```python
from build123d import *

# Parameters (mm, degrees)
F1_DEPTH = 22.5
F2_DEPTH = 8.5
F0_W     = 10
F0_H     = 50
F3_DEPTH = 17
F6_DEPTH = 14
F7_DEPTH = 18


with BuildPart() as f1:
    # F0 (on Front) → F1 (new body, symmetric)
    with BuildSketch(Plane.XZ):
        with BuildLine():
            Line((0, 15), (0, 25))
            ThreePointArc((0, 25), (-25, 0), (0, -25))
            Line((0, -25), (0, -15))
            ThreePointArc((0, -15), (-15, 0), (0, 15))
        make_face()
        with BuildLine():
            ThreePointArc((0, -25), (17.6776695297, -17.6776695297), (25, 0))
            ThreePointArc((25, 0), (17.6776695297, 17.6776695297), (0, 25))
            Line((0, 25), (0, 15))
            ThreePointArc((0, 15), (10.6066017178, 10.6066017178), (15, 0))
            ThreePointArc((15, 0), (10.6066017178, -10.6066017178), (0, -15))
            Line((0, -15), (0, -25))
        make_face()
    extrude(amount=F1_DEPTH, both=True)

    # F0 (on Front) → F2 (join, symmetric)
    with BuildSketch(Plane.XZ):
        with BuildLine():
            ThreePointArc((0, 25), (17.6776695297, 17.6776695297), (25, 0))
            ThreePointArc((25, 0), (17.6776695297, -17.6776695297), (0, -25))
            Line((0, -25), (70, -25))
            Line((70, -25), (70, 25))
            Line((70, 25), (0, 25))
        make_face()
    extrude(amount=F2_DEPTH, both=True)

    # F0 (on Front) → F3 (join, symmetric)
    with BuildSketch(Plane.XZ):
        with Locations((75, 0)):
            Rectangle(F0_W, F0_H)
    extrude(amount=F3_DEPTH, both=True)

    # F5 (on offset) → F6 (join)
    with BuildSketch(Plane.XZ.offset(17)):
        with BuildLine():
            Line((93.4168760482, 25), (70, 25))
            Line((70, 25), (70, -25))
            Line((70, -25), (93.4168760482, -25))
            ThreePointArc((93.4168760482, -25), (80, 0), (93.4168760482, 25))
        make_face()
    extrude(amount=F6_DEPTH)

    # F5 (on offset) → F7 (join)
    with BuildSketch(Plane.XZ.offset(17)):
        with BuildLine():
            Line((110, 25), (93.4168760482, 25))
            ThreePointArc((93.4168760482, 25), (80, 0), (93.4168760482, -25))
            Line((93.4168760482, -25), (110, -25))
            Line((110, -25), (110, -15))
            ThreePointArc((110, -15), (95, 0), (110, 15))
            Line((110, 15), (110, 25))
        make_face()
        with BuildLine():
            ThreePointArc((140, 0), (124.1863716546, 26.4338203685), (93.4168760482, 25))
            Line((93.4168760482, 25), (110, 25))
            Line((110, 25), (110, 15))
            ThreePointArc((110, 15), (120.6066017178, 10.6066017178), (125, 0))
            ThreePointArc((125, 0), (120.6066017178, -10.6066017178), (110, -15))
            Line((110, -15), (110, -25))
            Line((110, -25), (93.4168760482, -25))
            ThreePointArc((93.4168760482, -25), (124.1863716546, -26.4338203685), (140, 0))
        make_face()
    extrude(amount=F7_DEPTH)

    # F8: F1 across plane


with BuildPart() as f1_1:
    add(f1.part)
    add(f1.part.mirror(Plane.XZ))


solid = f1_1.part
```
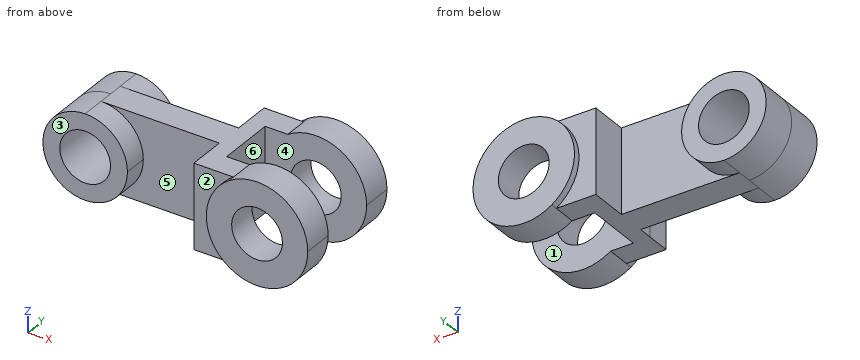
Geometry check sheet. Reference: the model listing, model coordinates, mm. Face numbers are marked on the shaded views. A direction names the side the tool comes from. Coordinates: 2 decimals unless noted, no trailing zeros. Order: outer loops, then holes, each group sorted by start corner. A loop starts at its lowest first (then second) coordinate and runs counter-clockwise, first axis right, second up. Notation, with made-up numbers: (-38.75, 66.5) - (-0.75, 66.5) arc R18 cw to (-0.75, 75.5) - close; hole circle Ø4 at (21, -27.75). An arc over 180 degrees is marked (long way). Answer as a JSON object with one key per item and string values. Group by question number.
Item 1: Sectioned sample at C-C, the plane y = 25.5. Record the cut outline in (x, z).
Item 2: Tool access check on the marked faces 1, 2 and 3. Record the directions out of +Z, -Z, +X, -X, +Y, -Y that give a thin tool (end or side, any length) a straight path to the whole face; none if there is none.
Item 3: Depth check by flat-ended pin: pin 1 Ø8 at (x, z) = (20, 16.5) entering from +Y; pin 2 Ø10 at (x, y) = (33, 3.5) entering from +Z; pin 3 Ø2 at (x, z) = (107, -12.5) entering from +Y; pin 4 Ø7 at (y, z) = (-12, -4.5) entering from -X. Enter the tip coordinate at first touch or a pass-through.
Item 4: Scan lines: probe 1 along Y at (x, z) = (99, 10.5); probe 2 along X at (y, z) = (-4, 0); probe 3 along Y at (x, z) = (29.5, -22). Record each from-to range of solid material in increasing order.
Item 5: Draft check along X on the marked faces 4, 5 and 6. Enter one of: +X half, -X half, draft (parallel to the pull), parting line (faces both ways), or undercut.
Item 6: Sectioned sample at B-B, the plane x = 110. Record the cut outline in (y, z).
Item 7: Sectioned sample at A-A, the plane y = -14.5. Record the cut outline in (x, z), and give its area (3 significant figures).
Item 8: Sectioned sample at D-D, the plane z = 4. Give the number of separate pieces and of enclosed holes in the cut face, and give its area (3 significant figures).
Resolved:
{
 "1": {"outline": "(70, -25) - (93.42, -25) arc R30 ccw (long way) to (93.42, 25) - (70, 25) - close; hole circle Ø30 at (110, 0)"},
 "2": {"face 1": "+Z, -Z, +X", "face 2": "-X, -Y", "face 3": "+Z, -Z, -X, -Y"},
 "3": {"pin 1": "y = 22.5", "pin 2": "z = 25", "pin 3": "through", "pin 4": "x = -24.98"},
 "4": {"probe 1": "-35 to -17, 17 to 35", "probe 2": "-25 to -15, 15 to 80", "probe 3": "-8.5 to 8.5"},
 "5": {"face 4": "draft", "face 5": "undercut", "face 6": "+X half"},
 "6": {"outline": "(-35, -30) - (-17, -30) - (-17, -15) - (-35, -15) - close; (-35, 15) - (-17, 15) - (-17, 30) - (-35, 30) - close; (17, -30) - (35, -30) - (35, -15) - (17, -15) - close; (17, 15) - (35, 15) - (35, 30) - (17, 30) - close"},
 "7": {"outline": "circle Ø50 at (0, 0); (70, -25) - (80, -25) - (80, 25) - (70, 25) - close; hole circle Ø30 at (0, 0)", "area": "1,760 mm^2"},
 "8": {"separate pieces": "4", "enclosed holes": "0", "area": "3,420 mm^2"}
}
